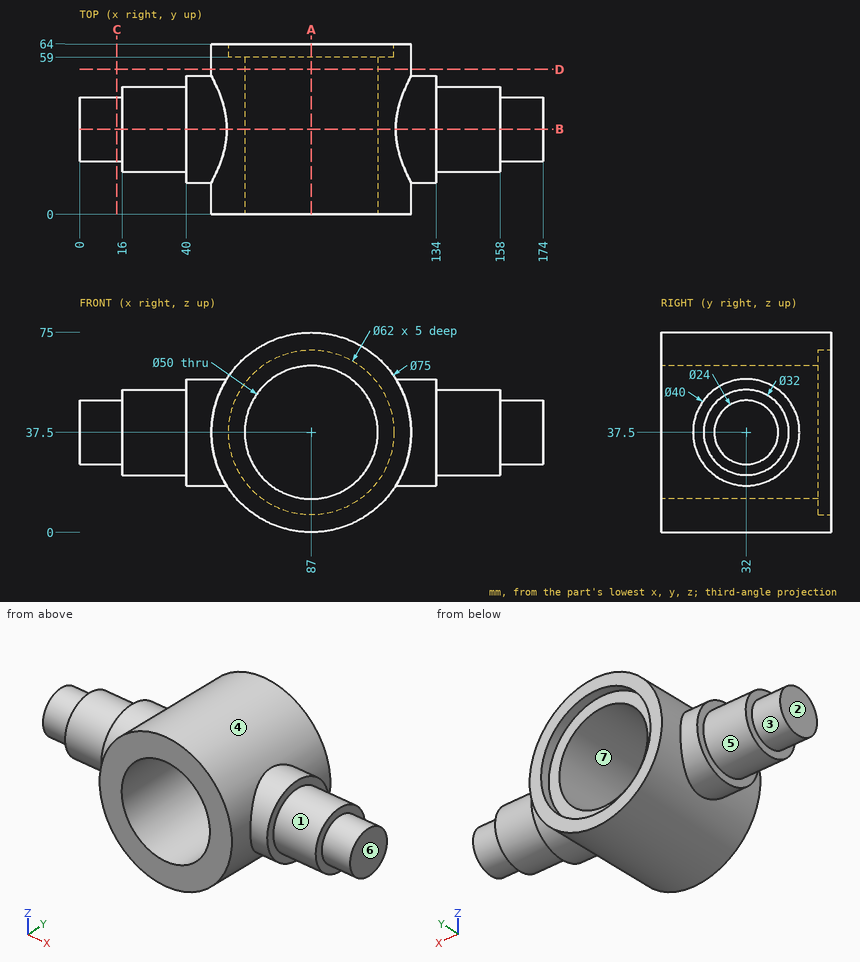
Part print with two shaded views. Sizes in mm from the minimum x, y, z corner. A direction names the side the tool comes from. Coordinates: 2 decimals unless noted, no trailing zeros. Write each loop counter-clockwise with the first axis right and the second up, starting at its lowest first coordinate (ties: lowest second). Pieces come first, ordered by that corner, then holes. Notation, with made-up numbers: (-0.75, 17) - (5.25, 17) arc R36 cw to (5.25, 52) - close; hole circle Ø2 at (64.25, 6.25). An arc over 180 degrees is marked (long way). One line per item, written item: value. Start each with the question number.
1. Mould opens along X. For the marked faces 4, 5, 6 and 7 say: released by +X, released by -X, zero draft, split by the parting line, or undercut.
2. Slice it at A-A (x = 87). Write the cut outline in (y, z).
3. Probe line 1 (X direction, y = 18, z = 37) (3 decimals); line 2 (X direction, y = 58.5, z = 37) (3 decimals); line 3 (Y direction, x = 104, z = 12). List the from-to ranges inside material, lowest first. Write a range as from..to.
4. Slice it at B-B (y = 32). Write the cut outline in (x, z).
5. Flat gauge pins, fed straight in: pin 1 (4 mm diameter, centred on x = 111.5, z = 41, fed in from +Y); pin 2 (5 mm diameter, centred on y = 34, z = 59.5, fed in from -X); pin 3 (3 mm diameter, centred on x = 120.5, y = 36, fed in from -Z). Where does each tip first touch, or does it go through?
6. Slice it at C-C (x = 14). Write the cut outline in (y, z), plus the area to 3 significant figures.
7. Slice it at D-D (y = 54.5). Write the cut outline in (x, z), plus the area to 3 significant figures.
8. Tool access for the marked faces 1, 2 and 3: list every direction of +Z, -Z, +X, -X, +Y, -Y with a clear straight run to the whole face (end or side of a thin tool).
Answers below:
1. face 4: split by the parting line
1. face 5: zero draft
1. face 6: released by +X
1. face 7: undercut
2. outline: (0, 0) - (64, 0) - (64, 6.5) - (59, 6.5) - (59, 12.5) - (0, 12.5) - close; (0, 62.5) - (59, 62.5) - (59, 68.5) - (64, 68.5) - (64, 75) - (0, 75) - close
3. line 1: x = 16..62.005, 111.995..158
3. line 2: x = 49.503..62.005, 111.995..124.497
3. line 3: y = 0..59
4. outline: (0, 25.5) - (16, 25.5) - (16, 21.5) - (40, 21.5) - (40, 17.5) - (55.28, 17.5) arc R37.5 ccw to (118.72, 17.5) - (134, 17.5) - (134, 21.5) - (158, 21.5) - (158, 25.5) - (174, 25.5) - (174, 49.5) - (158, 49.5) - (158, 53.5) - (134, 53.5) - (134, 57.5) - (118.72, 57.5) arc R37.5 ccw to (55.28, 57.5) - (40, 57.5) - (40, 53.5) - (16, 53.5) - (16, 49.5) - (0, 49.5) - close; hole circle Ø50 at (87, 37.5)
5. pin 1: stops at y = 59
5. pin 2: stops at x = 40
5. pin 3: stops at z = 17.66
6. outline: circle Ø24 at (32, 37.5)
6. area: 452 mm^2
7. outline: circle Ø75 at (87, 37.5); hole circle Ø50 at (87, 37.5)
7. area: 2,450 mm^2
8. face 1: +X
8. face 2: +Z, -Z, -X, +Y, -Y
8. face 3: -X
